Autodesk Inventor part; units mm, degrees
ref_plane "YZ Plane" through (0, 0, 0) normal (1, 0, 0) x (0, 1, 0)
ref_plane "XZ Plane" through (0, 0, 0) normal (0, 1, 0) x (-1, 0, 0)
ref_plane "XY Plane" through (0, 0, 0) normal (0, 0, 1) x (1, 0, 0)
sketch "スケッチ1" plane through (0, 0, 0) normal (0, 0, 1) x (1, 0, 0)
  line L0 (-30.25, 22.5) -> (30.25, 22.5)
  line L1 (30.25, 22.5) -> (30.25, -22.5)
  line L2 (30.25, -22.5) -> (-30.25, -22.5)
  line L3 (-30.25, -22.5) -> (-30.25, 22.5)
  line L4 (-25.25, 19.5) -> (25.25, 19.5) construction
  line L5 (25.25, 19.5) -> (25.25, -19.5) construction
  line L6 (25.25, -19.5) -> (-25.25, -19.5) construction
  line L7 (-25.25, -19.5) -> (-25.25, 19.5) construction
  line L8 (25.25, 19.5) -> (-25.25, -19.5) construction
  line L9 (-25.25, -17.6048) -> (-25.25, 19.5)
  line L10 (-25.25, 19.5) -> (22.7959, 19.5)
  line L11 (22.7959, 19.5) -> (-25.25, -17.6048)
  line L12 (-22.7959, -19.5) -> (25.25, -19.5)
  line L13 (25.25, -19.5) -> (25.25, 17.6048)
  line L14 (25.25, 17.6048) -> (-22.7959, -19.5)
  line L15 (-30.25, 20) -> (30.25, 20) construction
  line L16 (30.25, -20) -> (-30.25, -20) construction
  line L17 (30.25, 20) -> (30.25, -20) construction
  point P0 (0, 0)
  point P1 (0, 19.5)
  point P2 (0, 22.5)
  point P3 (25.25, 0)
  point P4 (30.25, 0)
  dimension "d0" = 5
  dimension "d1" = 3
  dimension "d2" = 1.5
  dimension "d3" = 40
  dimension "d4" = 2.5
  dimension "d19" = 60.5
extrude "押し出し1" add sketch "スケッチ1" along normal blind 5
sketch "スケッチ2" plane through (30.25, -22.5, 0) normal (1, 0, 0) x (0, 0, -1)
  line L0 (0, 45) -> (-5, 45)
  line L1 (-5, 0) -> (-5, 45)
  line L2 (0, 22.5) -> (-5, 22.5) construction
  point P0 (-2.5, 2.5)
  point P1 (-2.5, 22.5)
  point P2 (-2.5, 42.5)
  point P3 (-2.5, 45)
  dimension "d7" = 40
hole "穴1" at (30.25, -20, 2.5) at (30.25, 0, 2.5) at (30.25, 20, 2.5) direction (-1, 0, 0) diameter 2.459 depth 3
mirror "ミラー1" about plane through (0, 0, 0) normal (1, 0, 0) of "穴1"
fillet "フィレット1" radius 2 6 edges at (-22.7959, -19.5, 2.5) (-25.25, -17.6048, 2.5) (25.25, 17.6048, 2.5) (25.25, -19.5, 2.5) (-25.25, 19.5, 2.5) (22.7959, 19.5, 2.5)
equation "\"d3\" = d11_1"
properties part number "Link_front_diagonal" material "アルミニウム 2014-T4"
Input: part model. Units: mm. Frame: model coordinates. A direction names the side the tool comes from. Round coordinates to 2 decimals unless told otherwise and drop trailing zeros. Loops run counter-clockwise (first coordinate to the right, second up) from the corner with the lowest first, then second, coordinate; pieces in that order, holes last. Notation, with made-up numbers: (-25.75, 74) -> (-13.75, 74) arc R33 ccw to (-13.75, 104) -> close; hole circle Ø6 at (-28.5, -19). An arc over 180 degrees is marked (long way). One line per item, written item: value.
(1) Section D-D (y = 0). Return the cut outline in (x, z).
Geometry check:
outline: (-30.25, 0) -> (-25.25, 0) -> (-25.25, 5) -> (-30.25, 5) -> (-30.25, 3.73) -> (-27.25, 3.73) -> (-27.25, 1.27) -> (-30.25, 1.27) -> close; (-2.45, 0) -> (2.45, 0) -> (2.45, 5) -> (-2.45, 5) -> close; (25.25, 0) -> (30.25, 0) -> (30.25, 1.27) -> (27.25, 1.27) -> (27.25, 3.73) -> (30.25, 3.73) -> (30.25, 5) -> (25.25, 5) -> close
(2) Section B-B (x = -0.5). Return the cut outline in (y, z).
Geometry check:
outline: (-22.5, 0) -> (-19.5, 0) -> (-19.5, 5) -> (-22.5, 5) -> close; (-2.28, 0) -> (1.51, 0) -> (1.51, 5) -> (-2.28, 5) -> close; (19.5, 0) -> (22.5, 0) -> (22.5, 5) -> (19.5, 5) -> close
(3) Section C-C (z = 2.5). Give the number of separate pieces and of enclosed holes in the cut face, plus the area to 3 significant figures.
Geometry check:
separate pieces: 1
enclosed holes: 2
area: 918 mm2
(4) Mould query, pull axis Z, two halves, no side actions, for faces 4 (the face through (28.73, -18.8, 2.77)), 5 (the face through (-24.65, 18.93, 2.54)), 6 (the face through (-27.25, 0, 2)). Classes: pulls with the +Z half, pulls with the -Z half, needs draft (parallel to the pull), parting line crosses it, or undercut.
Geometry check:
face 4: undercut
face 5: needs draft
face 6: undercut
(5) Material intervals for line 1 (Y direction, x = -28.55, z = 2.5); line 2 (Z direction, x = -28.2, y = 0); line 3 (X direction, y = -13, z = 1.55), sorted ascending. Write a range as [from, to].
Geometry check:
line 1: [-22.5, -21.23], [-18.77, -1.23], [1.23, 18.77], [21.23, 22.5]
line 2: [0, 1.27], [3.73, 5]
line 3: [-30.25, -25.25], [-19.29, -14.38], [25.25, 30.25]
(6) Pin query (flat end, axial travel): pin 1 (1.2 mm diameter, centred on y = 20.5, z = 2.5, fed in from +X); pin 2 (2 mm diameter, centred on y = 0, z = 2.5, fed in from -X). Return the tip coordinate at first contact, or that it passes through.
Geometry check:
pin 1: x = 27.25
pin 2: x = -27.25
(7) Set-up query: faces 1 (the face through (-28.73, 18.8, 2.77)), 2 (the face through (2.22, -0.18, 2.46)), 3 (the face through (28.729, -0.369, 1.327)). Return all of +Z, -Z, +X, -X, +Y, -Y with unobstructed straight access to the full face (end or side cutting, diameter ignored); none if empty.
Geometry check:
face 1: -X
face 2: +Z, -Z
face 3: +X
(8) Section A-A (y = 10.5). Return the cut outline in (x, z), plus the area to 3 significant figures.
Geometry check:
outline: (-30.25, 0) -> (-25.25, 0) -> (-25.25, 5) -> (-30.25, 5) -> close; (11.14, 0) -> (16.05, 0) -> (16.05, 5) -> (11.14, 5) -> close; (25.25, 0) -> (30.25, 0) -> (30.25, 5) -> (25.25, 5) -> close
area: 74.5 mm2
